Can you work these out from the drawing? Everything is in mm from the part's minimum corner. A direction names the side the tool comes from. Round coordinates to 2 decimals unless told otherwise and drop trailing zeros. Order: outer loops, then holes, each group sorted by start corner. A loop starts at its lowest first (then second) coordinate and runs counter-clockwise, first axis right, second up. Notation, with made-up numbers: (35, 88) - (79, 88) arc R8 cw to (79, 97) - close; hole circle Ø8 at (-15.5, -30). An arc over 180 degrees is marked (long way). Answer as a JSON object with one key per item and string values.
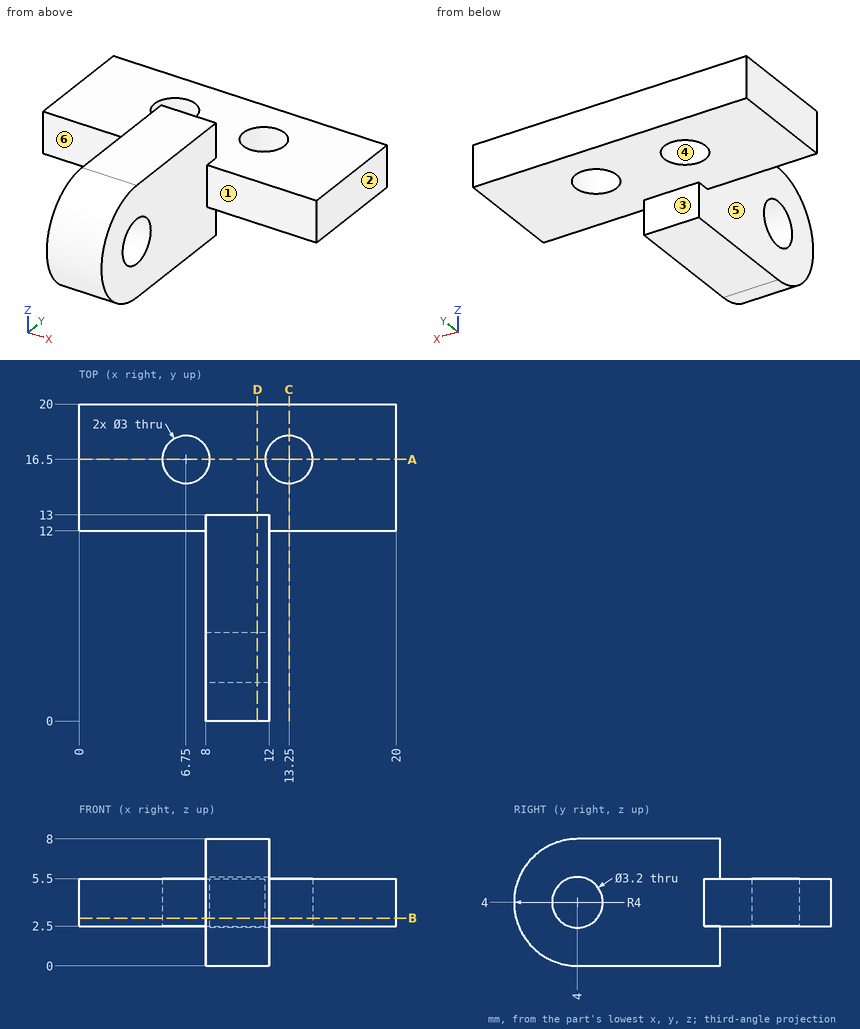
1. If I drill on L1, parallel to Y at x = 6.75, z = 4.3; L2, parallel to X at y = 15.5, z = 3; L3, parallel to Z at x = 10.75, y = 3.75, over which ranges is the centre line in solid material (lowest first)? Write a range as [from, to].
Responses:
{"L1": "[12, 15], [18, 20]", "L2": "[0, 5.63], [7.87, 12.13], [14.37, 20]", "L3": "[0.01, 2.42], [5.58, 7.99]"}
2. For the marked faces 1, 2 and 3, which set-ups out of +Z, -Z, +X, -X, +Y, -Y let a thin tool reach every point of the face, with its end or its side?
Responses:
{"face 1": "+Z, -Z, +X, -Y", "face 2": "+Z, -Z, +X, +Y, -Y", "face 3": "-Z, +X, -X, +Y"}
3. Imagine slicing it at A-A (y = 16.5). List the corners of the cut face in (x, z) for me.
Responses:
{"outline": "(0, 2.5) - (5.25, 2.5) - (5.25, 5.5) - (0, 5.5) - close; (8.25, 2.5) - (11.75, 2.5) - (11.75, 5.5) - (8.25, 5.5) - close; (14.75, 2.5) - (20, 2.5) - (20, 5.5) - (14.75, 5.5) - close"}
4. For P1, Ø1.8, axis at x = 6.75, y = 16.5, coming from the +Z side; P2, Ø4, axis at x = 10.5, y = 17, coming from the +Z side; P3, Ø2.5, axis at x = 17.5, z = 4, coming from the -Y side; P4, Ø9, axis at x = 14, y = 14.5, coming from the -Z side, each with a flat end and sliding along its axis, tell me the tip position at first contact or that it passes through.
Responses:
{"P1": "through", "P2": "z = 5.5", "P3": "y = 12", "P4": "z = 0"}
5. Imagine slicing it at C-C (x = 13.25). List the corners of the cut face in (y, z) for me, plus the area to 3 significant figures.
Responses:
{"outline": "(12, 2.5) - (15, 2.5) - (15, 5.5) - (12, 5.5) - close; (18, 2.5) - (20, 2.5) - (20, 5.5) - (18, 5.5) - close", "area": "15.0 mm2"}
6. Imagine slicing it at D-D (x = 11.25). List the corners of the cut face in (y, z) for me, plus the area to 3 significant figures.
Responses:
{"outline": "(4, 0) - (13, 0) - (13, 2.5) - (20, 2.5) - (20, 5.5) - (13, 5.5) - (13, 8) - (4, 8) arc R4 ccw to start; hole circle Ø3.2 at (4, 4)", "area": "110 mm2"}
7. Thinking about a two-plate mould opening in Y: for the marked faces 4, 5 and 6, which applies, pulls with the +Y half, pulls with the -Y half, needs draft (parallel to the pull), parting line crosses it, or undercut?
Responses:
{"face 4": "undercut", "face 5": "needs draft", "face 6": "pulls with the -Y half"}
8. Imagine slicing it at B-B (z = 3). List the corners of the cut face in (x, y) for me.
Responses:
{"outline": "(0, 12) - (8, 12) - (8, 5.25) - (12, 5.25) - (12, 12) - (20, 12) - (20, 20) - (0, 20) - close; (8, 0.13) - (12, 0.13) - (12, 2.75) - (8, 2.75) - close; hole circle Ø3 at (6.75, 16.5); hole circle Ø3 at (13.25, 16.5)"}
